from build123d import *

# Parameters (mm, degrees)
F1_DEPTH = 78.2
F3_DEPTH = 5


with BuildPart() as f1:
    # F0 (on Front) → F1 (new body)
    with BuildSketch(Plane.XZ):
        Polygon((0, 0), (-20, 0), (-20, -3.035), (20, -3.035), (20, 0.07), (0, 0.07), align=None)
    extrude(amount=F1_DEPTH)

    # F2 (on Top) → F3 (cut, symmetric)
    with BuildSketch(Plane.XY):
        Polygon((20, 0), (14.9, 0), (20, -5.1), align=None)
        Polygon((20, -78.2), (20, -73.1), (14.9, -78.2), align=None)
        Polygon((-20, -5.1), (-14.9, 0), (-20, 0), align=None)
        Polygon((-14.9, -78.2), (-20, -73.1), (-20, -78.2), align=None)
    extrude(amount=F3_DEPTH, both=True, mode=Mode.SUBTRACT)


solid = f1.part
Geometry check sheet. Reference: the model listing, model coordinates, mm. A direction names the side the tool comes from. Round coordinates to 2 decimals unless told otherwise and drop trailing zeros. Order: outer loops, then holes, each group sorted by start corner. A loop starts at its lowest first (then second) coordinate and runs counter-clockwise, first axis right, second up. Notation, with made-up numbers: M 0,72.25 L 59,72.25 A22 ccw 59,96.25 Z; hole C 24,6 d3. An arc over 180 degrees is marked long. Answer in a Markdown table with one row per item. Add a question column.
Item 1: Sectioned sample at B-B, the plane x = -11. Enter the section's corners in (y, z) (3 decimals), plus the area to 3 significant figures.
Item 2: Set-up check for faces 1 (the face through (17.5, -75.6, -1.5)), 2 (the face through (-10, -39, 0)): record each of +Z, -Z, +X, -X, +Y, -Y from which the full face is reachable in a straight line by a thin tool's end or side.
Item 3: Material ranges on L1, parallel to Z at x = -11, y = -15 (3 decimals); L2, parallel to Y at x = 16, z = -1.3; L3, parallel to Y at x = -18, z = -2, recorded low to high. Write a range as [from, to].
Item 4: Sectioned sample at A-A, the plane z = -1.75. Enter the section's corners in (x, y).
Item 5: Depth check by flat-ended pin: pin 1 Ø1.5 at (x, z) = (-4.5, -1.5) entering from +Y; pin 2 Ø5 at (x, y) = (-9.5, -45.5) entering from +Z. Enter the tip coordinate at first touch or a pass-through.
Filled in:
| question | item | result |
|---|---|---|
| 1 | outline | M -78.2,-3.035 L 0,-3.035 L 0,0 L -78.2,0 Z |
| 1 | area | 237 mm² |
| 2 | face 1 | +Z, -Z, +X, -Y |
| 2 | face 2 | +Z, -X, +Y, -Y |
| 3 | L1 | z = [-3.035, 0] |
| 3 | L2 | y = [-77.1, -1.1] |
| 3 | L3 | y = [-75.1, -3.1] |
| 4 | outline | M -20,-73.1 L -14.9,-78.2 L 14.9,-78.2 L 20,-73.1 L 20,-5.1 L 14.9,0 L -14.9,0 L -20,-5.1 Z |
| 5 | pin 1 | stops at y = 0 |
| 5 | pin 2 | stops at z = 0 |
